The listing builds one solid part. Answer for the finished solid, in the listing's coordinates (mm). Face numbers are marked on the shaded views. Give positions to 0.01 mm unless a question says otherwise; leave off trailing zeros. Write each loop counter-clockwise with the first axis right and the second up, starting at its lowest first coordinate (ties: lowest second). Pieces come first, ordered by that corner, then holes. Notation, with made-up numbers: (53.25, 35) - (59.25, 35) arc R13 cw to (59.25, 39) - close; hole circle Ø6 at (2, 21.5). An arc over 180 degrees is marked (long way). Answer as CSV lines item,"result". Start each with the question number.
(1) Find section A-A (z = 1499.5). Write down the section's boundary in (x, y), then the cut area to 3 significant figures.
(2) This flat-tipped pin is pushed along its axis until it touches: pin 1 Ø12 at (x, y) = (528, -183) entering from -Z. Where does it stop, or does it pass through?
(3) A straight line is drawn through the part: probe 1 along X at (y, z) = (-1051.5, 634.5). Find the intervals that lie inside material, in ascending order.
(4) For a pull along X with two mould halves and no side action, classify the marked faces 1 and 2 as pulls with the +X half, pulls with the -X half, needs draft (parallel to the pull), parting line crosses it, or undercut.
(5) Find section B-B (y = -517). State how many separate pieces and enclosed holes the cut face has, then the cut area to 3 significant figures.
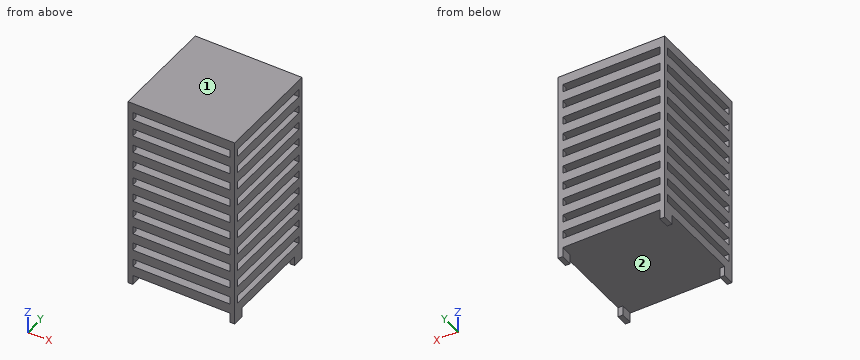
from build123d import *

# Parameters (mm, degrees)
F0_W     = 1000
F0_H     = 80
F1_DEPTH = 1100
F2_W     = 1000
F2_H     = 80
F2_W_2   = 860
F2_H_2   = 100
F3_DEPTH = 1100.001


with BuildPart() as f1:
    # F0 (on Front) → F1 (new body)
    with BuildSketch(Plane.XZ):
        Polygon((0, 2000), (0, 0), (50, 0), (50, 100), (1050, 100), (1050, 0), (1100, 0), (1100, 2000), align=None)
        with Locations((550, 240)):
            Rectangle(F0_W, F0_H, mode=Mode.SUBTRACT)
        with Locations((550, 420)):
            Rectangle(F0_W, F0_H, mode=Mode.SUBTRACT)
        with Locations((550, 600)):
            Rectangle(F0_W, F0_H, mode=Mode.SUBTRACT)
        with Locations((550, 780)):
            Rectangle(F0_W, F0_H, mode=Mode.SUBTRACT)
        with Locations((550, 960)):
            Rectangle(F0_W, F0_H, mode=Mode.SUBTRACT)
        with Locations((550, 1140)):
            Rectangle(F0_W, F0_H, mode=Mode.SUBTRACT)
        with Locations((550, 1320)):
            Rectangle(F0_W, F0_H, mode=Mode.SUBTRACT)
        with Locations((550, 1500)):
            Rectangle(F0_W, F0_H, mode=Mode.SUBTRACT)
        with Locations((550, 1680)):
            Rectangle(F0_W, F0_H, mode=Mode.SUBTRACT)
        with Locations((550, 1860)):
            Rectangle(F0_W, F0_H, mode=Mode.SUBTRACT)
    extrude(amount=F1_DEPTH)

    # F2 (on face) → F3 (cut, through all)
    with BuildSketch(Plane(origin=(0, 0, 0), x_dir=(0, -1, 0), z_dir=(-1, 0, 0))):
        with Locations((550, 1860)):
            Rectangle(F2_W, F2_H)
        with Locations((550, 1680)):
            Rectangle(F2_W, F2_H)
        with Locations((550, 1500)):
            Rectangle(F2_W, F2_H)
        with Locations((550, 1320)):
            Rectangle(F2_W, F2_H)
        with Locations((550, 1140)):
            Rectangle(F2_W, F2_H)
        with Locations((550, 960)):
            Rectangle(F2_W, F2_H)
        with Locations((550, 780)):
            Rectangle(F2_W, F2_H)
        with Locations((550, 600)):
            Rectangle(F2_W, F2_H)
        with Locations((550, 420)):
            Rectangle(F2_W, F2_H)
        with Locations((550, 240)):
            Rectangle(F2_W, F2_H)
        with Locations((550, 50)):
            Rectangle(F2_W_2, F2_H_2)
    extrude(amount=-F3_DEPTH, mode=Mode.SUBTRACT)


solid = f1.part
Result set:
1,outline,"(0, -1100) - (50, -1100) - (50, -1050) - (0, -1050) - close; (0, -50) - (50, -50) - (50, 0) - (0, 0) - close; (1050, -1100) - (1100, -1100) - (1100, -1050) - (1050, -1050) - close; (1050, -50) - (1100, -50) - (1100, 0) - (1050, 0) - close"
1,area,"10,000 mm^2"
2,pin 1,"z = 100"
3,probe 1,"0 to 50, 1050 to 1100"
4,face 1,"needs draft"
4,face 2,"undercut"
5,separate pieces,"11"
5,enclosed holes,"0"
5,area,"1,210,000 mm^2"
